Input: part model. Units: mm. Frame: model coordinates. Face numbers are marked on the shaded views. Round coordinates to 2 decimals unless told otherwise and drop trailing zeros. Order: outer loops, then holes, each group sorted by start corner. A loop starts at its lowest first (then second) coordinate and runs counter-clockwise, first axis right, second up. Notation, with made-up numbers: (34.25, 38) -> (89.25, 38) arc R17 cw to (89.25, 67) -> close; hole circle Ø5 at (-13.75, -24). An arc over 180 degrees is marked (long way). Use a Markdown table: item, result.
from build123d import *

# Parameters (mm, degrees)
F0_W     = 114.3
F0_H     = 266.7
F1_DEPTH = 25.4
F2_R     = 19.05
F3_DEPTH = 25.4


with BuildPart() as f1:
    # F0 (on Front) → F1 (new body)
    with BuildSketch(Plane.XZ):
        with Locations((-57.15, 133.35)):
            Rectangle(F0_W, F0_H)
    extrude(amount=F1_DEPTH)

    # F2 (on face) → F3 (cut)
    with BuildSketch(Plane.XZ.offset(25.4)):
        with BuildLine():
            Line((-25.4, 22.225), (-6.35, 22.225))
            ThreePointArc((-6.35, 22.225), (-25.4, 41.275), (-44.45, 22.225))
            Line((-44.45, 22.225), (-25.4, 22.225))
        make_face()
        with Locations((-76.2, 22.225)):
            Circle(F2_R)
        with BuildLine():
            ThreePointArc((-44.45, 22.225), (-25.4, 3.175), (-6.35, 22.225))
            Line((-6.35, 22.225), (-25.4, 22.225))
            Line((-25.4, 22.225), (-44.45, 22.225))
        make_face()
        with BuildLine():
            ThreePointArc((-69.85, 66.675), (-88.9, 85.725), (-107.95, 66.675))
            Line((-107.95, 66.675), (-88.9, 66.675))
            Line((-88.9, 66.675), (-69.85, 66.675))
        make_face()
        with BuildLine():
            ThreePointArc((-19.05, 66.675), (-38.1, 85.725), (-57.15, 66.675))
            ThreePointArc((-57.15, 66.675), (-38.1, 47.625), (-19.05, 66.675))
        make_face()
        with BuildLine():
            Line((-88.9, 66.675), (-107.95, 66.675))
            ThreePointArc((-107.95, 66.675), (-88.9, 47.625), (-69.85, 66.675))
            Line((-69.85, 66.675), (-88.9, 66.675))
        make_face()
        with Locations((-25.4, 111.125)):
            Circle(F2_R)
        with Locations((-76.2, 111.125)):
            Circle(F2_R)
        with Locations((-25.4, 200.025)):
            Circle(F2_R)
        with Locations((-76.2, 200.025)):
            Circle(F2_R)
        with Locations((-38.1, 155.575)):
            Circle(F2_R)
        with Locations((-88.9, 155.575)):
            Circle(F2_R)
        with Locations((-38.1, 244.475)):
            Circle(F2_R)
        with Locations((-88.9, 244.475)):
            Circle(F2_R)
    extrude(amount=-F3_DEPTH, mode=Mode.SUBTRACT)


solid = f1.part
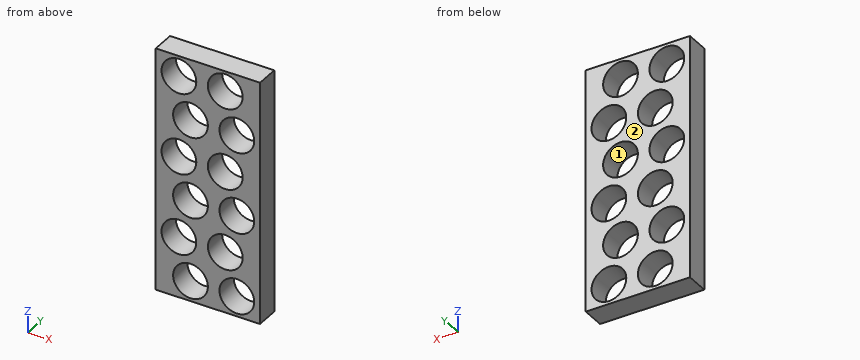
1) Pin query (flat end, axial travel): pin 1 Ø23 at (x, z) = (-25.4, 200.025) entering from -Y. Return the tip coordinate at first contact, or that it passes through.
Results found:
| item | result |
|---|---|
| pin 1 | passes through |
2) Cut plane A-A on x = -88.9. Return loops of the section in (y, z) (3 decimals), and give its area (3 significant figures).
Results found:
| item | result |
|---|---|
| outline | (-25.4, 0) -> (0, 0) -> (0, 8.026) -> (-25.4, 8.026) -> close; (-25.4, 36.424) -> (0, 36.424) -> (0, 47.625) -> (-25.4, 47.625) -> close; (-25.4, 85.725) -> (0, 85.725) -> (0, 96.926) -> (-25.4, 96.926) -> close; (-25.4, 125.324) -> (0, 125.324) -> (0, 136.525) -> (-25.4, 136.525) -> close; (-25.4, 174.625) -> (0, 174.625) -> (0, 185.826) -> (-25.4, 185.826) -> close; (-25.4, 214.224) -> (0, 214.224) -> (0, 225.425) -> (-25.4, 225.425) -> close; (-25.4, 263.525) -> (0, 263.525) -> (0, 266.7) -> (-25.4, 266.7) -> close |
| area | 1,710 mm² |
3) Cut plane C-C on x = -63.5. Return loops of the section in (y, z).
Results found:
| item | result |
|---|---|
| outline | (-25.4, 0) -> (0, 0) -> (0, 8.03) -> (-25.4, 8.03) -> close; (-25.4, 36.42) -> (0, 36.42) -> (0, 96.93) -> (-25.4, 96.93) -> close; (-25.4, 125.32) -> (0, 125.32) -> (0, 185.83) -> (-25.4, 185.83) -> close; (-25.4, 214.22) -> (0, 214.22) -> (0, 266.7) -> (-25.4, 266.7) -> close |
4) Pull-direction query (Z, two-part tool) for the marked faces 1 and 2; classes: +Z half, -Z half, draft (parallel to the pull), parting line (faces both ways), or undercut.
Results found:
| item | result |
|---|---|
| face 1 | undercut |
| face 2 | draft |
5) Cut plane B-B on z = 74.5. Return loops of the section in (x, y), and give its area (3 significant figures).
Results found:
| item | result |
|---|---|
| outline | (-114.3, -25.4) -> (-106.27, -25.4) -> (-106.27, 0) -> (-114.3, 0) -> close; (-71.53, -25.4) -> (-55.47, -25.4) -> (-55.47, 0) -> (-71.53, 0) -> close; (-20.73, -25.4) -> (0, -25.4) -> (0, 0) -> (-20.73, 0) -> close |
| area | 1,140 mm² |
6) Line query: L1, parallel to X at y = -18, z = 28.5; L2, parallel to X at y = -19.75, z = 213.5; L3, parallel to Z at x = -60, y = -7. Output: solid intervals per line, ascending. Write a range as [from, to].
Results found:
| item | result |
|---|---|
| L1 | x = [-114.3, -94.19], [-58.21, -43.39], [-7.41, 0] |
| L2 | x = [-114.3, -89.67], [-62.73, -38.87], [-11.93, 0] |
| L3 | z = [0, 12.2], [32.25, 101.1], [121.15, 190], [210.05, 266.7] |
7) Cut plane D-D on y = -10.5. Count the separate pieces of the cut face and the enclosed holes in it, and give its area (3 significant figures).
Results found:
| item | result |
|---|---|
| separate pieces | 1 |
| enclosed holes | 12 |
| area | 16,800 mm² |
